Verification items for the finished model (mm, model axes). A direction names the side the tool comes from. Coordinates: 2 decimals unless noted, no trailing zeros. One line per item, written item: value. Start each with the question number.
(1) Set-up check for faces 4 (the face through (15.324, 13.882, 7.041)), 5 (the face through (-15.885, 16.103, 10.65)), 6 (the face through (2.7, -12.15, 5.58)): record each of +Z, -Z, +X, -X, +Y, -Y from which the full face is reachable in a straight line by a thin tool's end or side.
(2) Thickness scan on probe 1 along Y at (x, z) = (10, 5); probe 2 along Z at (x, y) = (-24, 25); probe 3 along Y at (x, z) = (-9, 2.5). Record the ranges inside material, lowest first. Write a range as [from, to].
(3) Gauge pin test, flat ends, axial feed: P1, Ø5.5, axis at x = -12.5, y = 14.5, coming from the +Z side; P2, Ø23, axis at x = -4.5, y = -14.5, coming from the -Z side; P3, Ø5.5, axis at x = 13, y = -14, coming from the +Z side. Record the tip position at first contact, or that the pin passes through.
(4) Draft check along X on faces 1 (the face through (-11.04, -49.716, 5.009)), 2 (the face through (19, -34, 0)), 3 (the face through (15, -12, 9.195)). Enter one of: +X half, -X half, draft (parallel to the pull), parting line (faces both ways), or undercut.
```python
from build123d import *

# Parameters (mm, degrees)
SKETCH1_R                                     = 50.927
BOSS_EXTRUDE1_DEPTH                           = 12.7
W_0_386_DIAMETER_HOLE1_D                      = 9.8044
W_0_386_DIAMETER_HOLE1_CSINK_D                = 11.0744
W_0_386_DIAMETER_HOLE1_CSINK_ANGLE            = 90
CBORE_FOR_6_SOCKET_HEAD_CAP_SCREW1_AT_2_COUNT = 2
CBORE_FOR_6_SOCKET_HEAD_CAP_SCREW1_AT_2_PITCH = 38.1
CBORE_FOR_6_SOCKET_HEAD_CAP_SCREW1_AT_3_COUNT = 2
CBORE_FOR_6_SOCKET_HEAD_CAP_SCREW1_AT_3_PITCH = 26.940768363
CBORE_FOR_6_SOCKET_HEAD_CAP_SCREW1_AT_4_COUNT = 2
CBORE_FOR_6_SOCKET_HEAD_CAP_SCREW1_AT_4_PITCH = 26.940768363
FILLET1_R                                     = 2.54
SKETCH7_R                                     = 15.9385
SKETCH7_R_2                                   = 12.446
CUT_EXTRUDE2_DEPTH                            = 6.35
SKETCH6_R                                     = 38.1
CUT_EXTRUDE1_DEPTH                            = 4.826


with BuildPart() as part:
    # Sketch1 → Boss-Extrude1 (new body)
    with BuildSketch(Plane.XY):
        Circle(SKETCH1_R)
    extrude(amount=BOSS_EXTRUDE1_DEPTH)

    # W (0.386) Diameter Hole1 (through all)
    with Locations(Plane.XY.offset(12.7)):
        with Locations((0, 0)):
            CounterSinkHole(W_0_386_DIAMETER_HOLE1_D / 2, W_0_386_DIAMETER_HOLE1_CSINK_D / 2, counter_sink_angle=W_0_386_DIAMETER_HOLE1_CSINK_ANGLE)

    # Sketch5 → CBORE for #6 Socket Head Cap Screw1 (revolve, cut)
    with BuildSketch(Plane(origin=(13.470384182, 13.470384182, 12.7), x_dir=(0, -1, 0), z_dir=(1, 0, 0))):
        Polygon((0, 0), (0, 12.7), (1.89865, 12.7), (1.89865, 3.5052), (3.57251, 3.5052), (3.57251, 0.635), (4.20751, 0), align=None)
    cbore_for_6_socket_head_cap_screw1 = revolve(axis=Axis((13.470384182, 13.470384182, 19.05), (0, 0, -1)), mode=Mode.SUBTRACT)

    # CBORE for #6 Socket Head Cap Screw1 at 2: CBORE for #6 Socket Head Cap Screw1 ×2
    with Locations(*[Vector(-0.707106781, -0.707106781, 0) * (i * CBORE_FOR_6_SOCKET_HEAD_CAP_SCREW1_AT_2_PITCH) for i in range(1, CBORE_FOR_6_SOCKET_HEAD_CAP_SCREW1_AT_2_COUNT)]):
        add(cbore_for_6_socket_head_cap_screw1, mode=Mode.SUBTRACT)

    # CBORE for #6 Socket Head Cap Screw1 at 3: CBORE for #6 Socket Head Cap Screw1 ×2
    with Locations(*[(-i * CBORE_FOR_6_SOCKET_HEAD_CAP_SCREW1_AT_3_PITCH, 0, 0) for i in range(1, CBORE_FOR_6_SOCKET_HEAD_CAP_SCREW1_AT_3_COUNT)]):
        add(cbore_for_6_socket_head_cap_screw1, mode=Mode.SUBTRACT)

    # CBORE for #6 Socket Head Cap Screw1 at 4: CBORE for #6 Socket Head Cap Screw1 ×2
    with Locations(*[(0, -i * CBORE_FOR_6_SOCKET_HEAD_CAP_SCREW1_AT_4_PITCH, 0) for i in range(1, CBORE_FOR_6_SOCKET_HEAD_CAP_SCREW1_AT_4_COUNT)]):
        add(cbore_for_6_socket_head_cap_screw1, mode=Mode.SUBTRACT)

    # Fillet1
    fillet1_edges = [part.edges().sort_by_distance(p)[0] for p in [
        (-50.927, 0, 12.7),
    ]]
    fillet(fillet1_edges, radius=FILLET1_R)

    # Sketch7 → Cut-Extrude2 (cut)
    with BuildSketch(Plane(origin=(0, 0, 0), x_dir=(-1, 0, 0), z_dir=(0, 0, -1))):
        Circle(SKETCH7_R)
        Circle(SKETCH7_R_2, mode=Mode.SUBTRACT)
    extrude(amount=-CUT_EXTRUDE2_DEPTH, mode=Mode.SUBTRACT)

    # Sketch6 → Cut-Extrude1 (cut)
    with BuildSketch(Plane(origin=(0, 0, 0), x_dir=(-1, 0, 0), z_dir=(0, 0, -1))):
        Circle(SKETCH6_R)
    extrude(amount=-CUT_EXTRUDE1_DEPTH, mode=Mode.SUBTRACT)


solid = part.part
```
Responses:
1. face 4: +Z, -Z
1. face 5: +Z
1. face 6: -Z
2. probe 1: y = [-49.94, -12.41], [-7.41, 7.41], [12.41, 49.94]
2. probe 2: z = [4.83, 12.7]
2. probe 3: y = [-50.13, -37.02], [37.02, 50.13]
3. P1: stops at z = 12.66
3. P2: stops at z = 4.83
3. P3: stops at z = 9.19
4. face 1: parting line
4. face 2: draft
4. face 3: undercut
